Can you work these out from the drawing? Everything is in mm from the part's minimum corner. A direction names the side the tool comes from. Round coordinates to 2 decimals unless told otherwise and drop trailing zeros. Write each loop counter-clockwise with the first axis right and the second up, starting at its lowest first coordinate (ties: lowest second). Pieces come first, ordered by that corner, then holes. Notation, with made-up numbers: (-21.75, 37.25) - (-12.75, 37.25) arc R8 ccw to (-12.75, 52.25) - close; hole circle Ø9 at (-10, 48.5). An arc over 180 degrees is marked (long way). Write each question's results on one line, items separated by ' | '. Start each with the question number.
(1) Imagine slicing it at C-C on y = 140.5. Write out the boundary of the cut face in (x, z).
(2) On a 3-axis mill with a long thin cutter (end or side, diameter ignored), from which of +Z, -Z, +X, -X, +Y, -Y can I reach the whole of each face in a straight line? I mean the marked faces 1 and 2. Say none if no direction works.
(3) Imagine slicing it at A-A on y = 114.3. Write out the boundary of the cut face in (x, z).
(4) Imagine slicing it at D-D on z = 14. Write out the boundary of the cut face in (x, y).
(5) Imagine slicing it at B-B on x = 53. Write out the boundary of the cut face in (y, z), then the cut area to 3 significant figures.
(6) Thinking about a two-plate mould opening in Z: for the marked faces 3, 4, 5 and 6, which applies, +Z half, -Z half, draft (parallel to the pull), parting line (faces both ways), or undercut?
(7) Please list where these lines run through material, in increasing order: line 1 (Z direction, x = 20, y = 114.3); line 2 (Z direction, x = 32, y = 114.3); line 3 (Y direction, x = 26, z = 31). Write a range as [from, to].
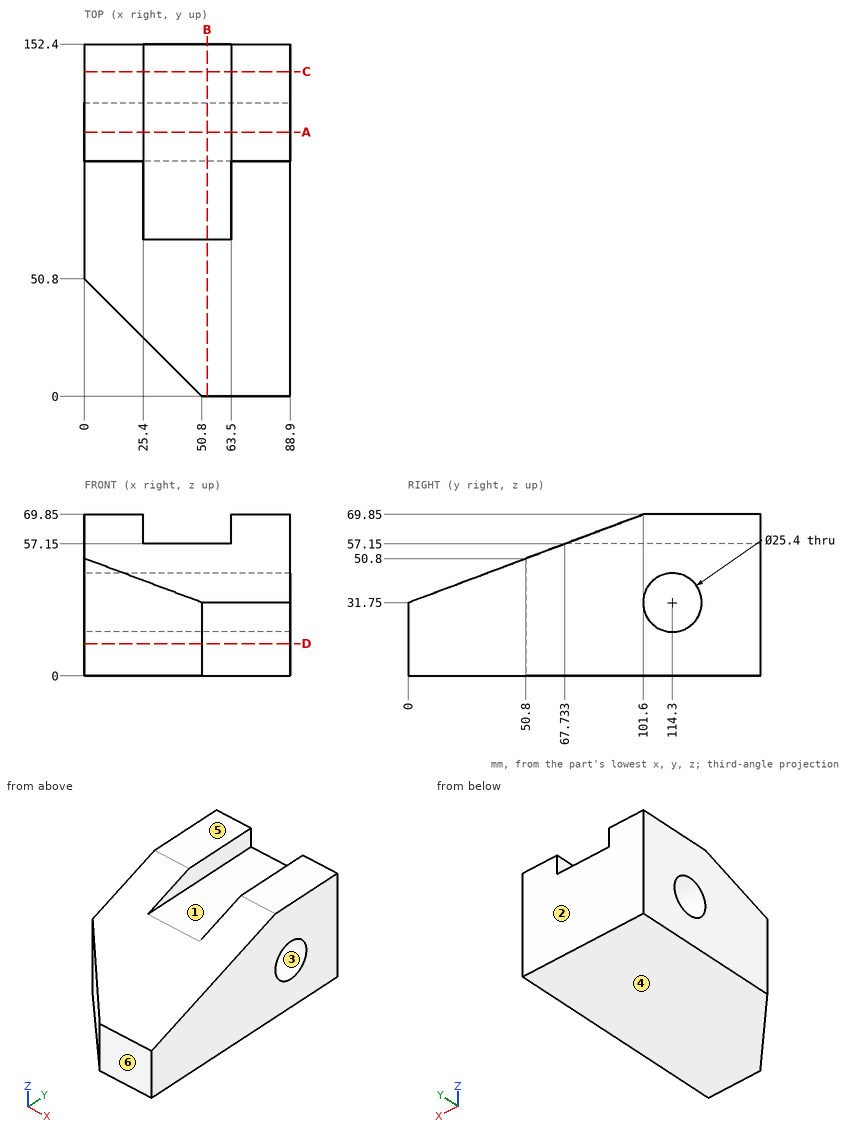
Response:
1) outline: (0, 0) - (88.9, 0) - (88.9, 69.85) - (63.5, 69.85) - (63.5, 57.15) - (25.4, 57.15) - (25.4, 69.85) - (0, 69.85) - close
2) face 1: +Z, +Y, -Y | face 2: +Z, -Z, +X, -X, +Y
3) outline: (0, 0) - (88.9, 0) - (88.9, 19.05) - (0, 19.05) - close; (0, 44.45) - (88.9, 44.45) - (88.9, 69.85) - (63.5, 69.85) - (63.5, 57.15) - (25.4, 57.15) - (25.4, 69.85) - (0, 69.85) - close
4) outline: (0, 50.8) - (50.8, 0) - (88.9, 0) - (88.9, 152.4) - (0, 152.4) - close
5) outline: (0, 0) - (152.4, 0) - (152.4, 57.15) - (67.73, 57.15) - (0, 31.75) - close; hole circle Ø25.4 at (114.3, 31.75) | area: 7,340 mm²
6) face 3: undercut | face 4: -Z half | face 5: +Z half | face 6: draft
7) line 1: [0, 19.05], [44.45, 69.85] | line 2: [0, 19.05], [44.45, 57.15] | line 3: [24.8, 101.62], [126.98, 152.4]
